from build123d import *

# Parameters (mm, degrees)
SKETCH_1_W          = 322.1
SKETCH_1_H          = 152.4
EXTRUDE_1_DEPTH     = 15
CUT_EXTRUDE_START   = 152.4
SKETCH_2_R          = 1
CUT_EXTRUDE_1_DEPTH = 50.8
CUT_EXTRUDE_2_DEPTH = 357.649926398


with BuildPart() as part:
    # 草图1 → 凸台-拉伸1 (new body)
    with BuildSketch(Plane.XY):
        with Locations((161.05, 76.2)):
            Rectangle(SKETCH_1_W, SKETCH_1_H)
    extrude(amount=EXTRUDE_1_DEPTH)

    # 草图2 → 切除-拉伸1 (cut)
    with BuildSketch(Plane(origin=(0, 0, 0), x_dir=(1, 0, 0), z_dir=(0, 1, 0)).offset(CUT_EXTRUDE_START)):
        with Locations(Location((161.05, -7.5, 0), (0, 0, 90))):
            Circle(SKETCH_2_R)
        with Locations(Location((211.85, -7.5, 0), (0, 0, 90))):
            Circle(SKETCH_2_R)
        with Locations(Location((262.65, -7.5, 0), (0, 0, 90))):
            Circle(SKETCH_2_R)
        with Locations(Location((110.25, -7.5, 0), (0, 0, 90))):
            Circle(SKETCH_2_R)
        with Locations(Location((59.45, -7.5, 0), (0, 0, 90))):
            Circle(SKETCH_2_R)
    extrude(amount=-CUT_EXTRUDE_1_DEPTH, mode=Mode.SUBTRACT)

    # 草图3 → 切除-拉伸2 (cut, through all)
    with BuildSketch(Plane.ZY):
        Polygon((0, 152.4), (15, 137.4), (15, 152.4), align=None)
    extrude(amount=-CUT_EXTRUDE_2_DEPTH, mode=Mode.SUBTRACT)


solid = part.part
Model file for the job. Use its own axes, mm. Round coordinates to 2 decimals unless told otherwise and drop trailing zeros. Order: outer loops, then holes, each group sorted by start corner. A loop starts at its lowest first (then second) coordinate and runs counter-clockwise, first axis right, second up. Notation, with made-up numbers: M 14.5,1.25 L 48.5,1.25 A27 ccw 48.5,26.25 Z; hole C -11.5,63.5 d9. An arc over 180 degrees is marked long. Write each question's results on one line, items separated by ' | '. Start each with the question number.
(1) Drop flat-ended pins along their axis: pin 1 (1 mm diameter, centred on x = 59.5, z = 7.5, fed in from +Y); pin 2 (6 mm diameter, centred on y = 61.5, z = 5.5, fed in from -X); pin 3 (3 mm diameter, centred on x = 110.25, z = 7.5, fed in from +Y); pin 4 (8 mm diameter, centred on x = 246.5, z = 6, fed in from +Y). Give the stop position or say it passes through.
(2) Saw through at B-B, the plane x = 268.5. Give the cut face in (y, z).
(3) Probe probe 1 along X at (y, z) = (133, 7.5); probe 2 along Z at (x, y) = (110.25, 115); probe 3 along Z at (x, y) = (59, 113). List the from-to ranges inside material, lowest first. Write a range as from..to.
(4) Saw through at A-A, the plane z = 4. Give the cut face in (x, y).
Established:
1) pin 1: stops at y = 101.6 | pin 2: stops at x = 0 | pin 3: stops at y = 146.4 | pin 4: stops at y = 150.4
2) outline: M 0,0 L 152.4,0 L 137.4,15 L 0,15 Z
3) probe 1: x = 0..58.45, 60.45..109.25, 111.25..160.05, 162.05..210.85, 212.85..261.65, 263.65..322.1 | probe 2: z = 0..6.5, 8.5..15 | probe 3: z = 0..6.61, 8.39..15
4) outline: M 0,0 L 322.1,0 L 322.1,148.4 L 0,148.4 Z
